Model file for the job. Use its own axes, mm. A direction names the side the tool comes from. Coordinates: 2 decimals unless noted, no trailing zeros. Write each loop counter-clockwise with the first axis right and the second up, starting at its lowest first coordinate (ties: lowest second). Pieces come first, ordered by that corner, then holes. Notation, with made-up numbers: (86, 25.25) -> (138, 25.25) arc R20 cw to (138, 29.25) -> close; hole circle Ø5 at (53, 47). An arc over 180 degrees is marked (long way). Write item = value, one per line. Start each with the question number.
from build123d import *

# Parameters (mm, degrees)
F1_DEPTH = 104
F2_T     = -12
F3_W     = 12
F3_H     = 196
F3_H_2   = 146
F4_DEPTH = 92
F5_W     = 76
F5_H     = 12
F5_W_2   = 89.8888036609
F5_W_3   = 87.8371410072
F6_DEPTH = 92


with BuildPart() as f1:
    # F0 (on Front) → F1 (new body)
    with BuildSketch(Plane.XZ):
        Polygon((-189.3542973706, 100), (-189.3542973706, -170), (110.6457026294, -170), (110.6457026294, 0), (10.6457026294, 0), (10.6457026294, 50), (-89.3542973706, 50), (-89.3542973706, 100), align=None)
    extrude(amount=F1_DEPTH)

    # F2
    f2_openings = [f1.faces().sort_by_distance(p)[0] for p in [
        (-54.505813, -104, -56.212121),
    ]]
    offset(amount=F2_T, openings=f2_openings, kind=Kind.INTERSECTION)

    # F3 (on face) → F4 (join)
    with BuildSketch(Plane.XZ.offset(12)):
        with Locations((-95.3542973706, -60)):
            Rectangle(F3_W, F3_H)
        with Locations((4.6457026294, -85)):
            Rectangle(F3_W, F3_H_2)
    extrude(amount=F4_DEPTH)

    # F5 (on face) → F6 (join)
    with BuildSketch(Plane.XZ.offset(12)):
        with Locations((-139.3542973706, -8.0260672197)):
            Rectangle(F5_W, F5_H)
        with Locations((-44.9444018304, -57.5752230883)):
            Rectangle(F5_W_2, F5_H)
        with Locations((54.2541909963, -95.0186225176)):
            Rectangle(F5_W_3, F5_H)
    extrude(amount=F6_DEPTH)


solid = f1.part
(1) Mould opens along Z. For faces 4 (the face through (-189.354, -51, -33)), 5 (the face through (-41, -51, -170)), 6 (the face through (-140, -57, -2.026)) say: released by +Z, released by -Z, zero draft, split by the parting line, or undercut.
(2) Saw through at D-D (z = -93.5). Give the cut face in (x, y), then the cut area to 3 significant figures.
(3) 3-axis set-ups, long thin cutter, end or side, ignore diameter. For faces 1 (the face through (10.646, -51, 25)), 2 (the face through (-177.354, -57, 44)), 3 (the face through (110.646, -51, -86)): which of +Z, -Z, +X, -X, +Y, -Y reach the whole face in a straight line?
(4) Saw through at A-A (y = -86.5). State how many separate pieces and enclosed holes the cut face has, then the cut area to 3 significant figures.
(5) Saw through at C-C (z = -56.5). Give the cut face in (x, y), then the cut area to 3 significant figures.
(6) Drill centre lines: line 1 along Z through (x, y) = (-138.5, -40); line 2 along Z through (x, y) = (-87, -70); line 3 along X through (y, z) = (-27, 32.5). Where is each one in solid material? Low to high.
(7) Saw through at B-B (x = -130.5). Give the cut face in (y, z).
Returned:
q1.face_4 = zero draft
q1.face_5 = released by -Z
q1.face_6 = undercut
q2.outline = (-189.35, -104) -> (-177.35, -104) -> (-177.35, -12) -> (-101.35, -12) -> (-101.35, -104) -> (-89.35, -104) -> (-89.35, -12) -> (-1.35, -12) -> (-1.35, -104) -> (98.17, -104) -> (98.17, -12) -> (98.65, -12) -> (98.65, -104) -> (110.65, -104) -> (110.65, 0) -> (-189.35, 0) -> close
q2.area = 16,100 mm2
q3.face_1 = +Z, +X, +Y, -Y
q3.face_2 = -Y
q3.face_3 = +Z, -Z, +X, +Y, -Y
q4.separate_pieces = 1
q4.enclosed_holes = 5
q4.area = 20,200 mm2
q5.outline = (-189.35, -104) -> (-177.35, -104) -> (-177.35, -12) -> (-101.35, -12) -> (-101.35, -104) -> (10.65, -104) -> (10.65, -12) -> (98.65, -12) -> (98.65, -104) -> (110.65, -104) -> (110.65, 0) -> (-189.35, 0) -> close
q5.area = 16,100 mm2
q6.line_1 = -170 to -158, -14.03 to -2.03, 88 to 100
q6.line_2 = -170 to -158, -63.58 to -51.58, 38 to 50
q6.line_3 = -189.35 to -177.35, -101.35 to -89.35, -1.35 to 10.65
q7.outline = (-104, -170) -> (0, -170) -> (0, 100) -> (-104, 100) -> (-104, 88) -> (-12, 88) -> (-12, -2.03) -> (-104, -2.03) -> (-104, -14.03) -> (-12, -14.03) -> (-12, -158) -> (-104, -158) -> close
